Design review of the part built by this model. Coordinates are the model's own, in mm. A direction names the side the tool comes from. Round coordinates to 2 decimals unless told otherwise and drop trailing zeros. Write each loop counter-clockwise with the first axis right and the second up, starting at its lowest first coordinate (ties: lowest second). Pieces come first, ordered by that corner, then holes. Notation, with made-up numbers: (4.25, 17) - (55.25, 17) arc R31 ccw to (55.25, 46) - close; hole circle Ø8 at (88.25, 85). An arc over 180 degrees is marked (long way). Use one line per item in the form item = value.
```python
from build123d import *


with BuildPart() as part:
    # Sketch1 → Revolve1 (revolve)
    with BuildSketch(Plane.XY, mode=Mode.PRIVATE) as revolve1_sk:
        with BuildLine():
            Line((0, 0), (95, 0))
            Line((95, 0), (95, 5))
            Line((95, 5), (120, 5))
            Line((120, 5), (120, 12))
            Line((120, 12), (117, 15))
            Line((117, 15), (100, 15))
            Line((100, 15), (95, 20))
            Line((95, 20), (20, 20))
            ThreePointArc((20, 20), (5.857864376, 14.142135624), (0, 0))
        make_face()
    revolve(revolve1_sk.sketch.rotate(Axis((0, 0, 0), (1, 0, 0)), 90), axis=Axis((0, 0, 0), (1, 0, 0)))


solid = part.part
```
Q1. We need section A-A on z = 0. Write out the cut boundary in (x, y).
Calculated:
outline = (20, -20) - (95, -20) - (100, -15) - (117, -15) - (120, -12) - (120, -5) - (95, -5) - (95, 5) - (120, 5) - (120, 12) - (117, 15) - (100, 15) - (95, 20) - (20, 20) arc R20 ccw to start
Q2. For P1, Ø2, axis at x = 72, y = -7, coming from the +Z side; P2, Ø5, axis at x = 31, z = -1, coming from the +Y side; P3, Ø4, axis at x = 94.5, y = 9, coming from the -Z side (3 decimals), all flat-tipped, find the tip position at first contact; note any pin that passes through.
Calculated:
P1 = 19.08
P2 = 20
P3 = -18.735
Q3. Machinability: for faces 1 (the cylindrical face through (56.98, -0.88, -19.98)), 2 (the cylindrical face through (108, 0, -5)), which of the approach directions +Z, -Z, +X, -X, +Y, -Y give a long, thin tool a straight path to every point of the face, cutting with its end or side? Answer none if there is none.
Calculated:
face_1 = +X, -X
face_2 = +X
Q4. We need section C-C on x = 97.5. Write out the cut boundary in (y, z), then the cut area to 3 significant figures.
Calculated:
outline = circle Ø35 at (0, 0); hole circle Ø10 at (0, 0)
area = 884 mm2
Q5. Draft analysis for pull direction Z (two halves, no side actions). For faces 3 (the flat face through (120, -0.2, -5.2)), 4 (the conical face through (99.687, -4.6, 14.606)), 5 (the flat face through (95, 0, 0)), state which applies: released by +Z, released by -Z, zero draft, split by the parting line, or undercut.
Calculated:
face_3 = zero draft
face_4 = split by the parting line
face_5 = undercut
Q6. We need section D-D on x = 83. Write out the cut boundary in (y, z), then the cut area to 3 significant figures.
Calculated:
outline = circle Ø40 at (0, 0)
area = 1,260 mm2
Q7. To check wall thickness, follow line 1 along Y through (x, z) = (100.25, 0); line 2 along X through (y, z) = (-12, 1); line 3 along Y through (x, z) = (59, 11). State the ranges of each line that lie inside material, in increasing order. Write a range as from..to.
Calculated:
line_1 = -15..-5, 5..15
line_2 = 4.03..119.96
line_3 = -16.7..16.7
